Autodesk Inventor part; units mm, degrees
ref_plane "YZ Plane" through (0, 0, 0) normal (1, 0, 0) x (0, 1, 0)
ref_plane "XZ Plane" through (0, 0, 0) normal (0, 1, 0) x (-1, 0, 0)
ref_plane "XY Plane" through (0, 0, 0) normal (0, 0, 1) x (1, 0, 0)
sketch "Sketch1" plane through (0, 0, 0) normal (0, 0, 1) x (1, 0, 0)
  circle A0 centre (-18.3043, -1.4966) radius 1.7
  circle A1 centre (18.6957, -1.4966) radius 1.7
  circle A2 centre (18.6957, 6.5034) radius 1.7
  circle A3 centre (-18.3043, 6.5034) radius 1.7
  circle A4 centre (11.6957, 6.5034) radius 1.7
  arc A5 (22.6957, 8.5034) -> (18.6957, 12.5034) centre (18.6957, 8.5034) ccw
  line L0 (4.8957, 12.5034) -> (18.6957, 12.5034)
  arc A6 (4.8957, 12.5034) -> (2.8957, 10.5034) centre (4.8957, 10.5034) ccw
  line L1 (2.8957, 6.5034) -> (2.8957, 10.5034)
  arc A7 (-9.5043, 6.5034) -> (2.8957, 6.5034) centre (-3.3043, 6.5034) ccw
  line L2 (-9.5043, 10.5034) -> (-9.5043, 6.5034)
  arc A8 (-9.5043, 10.5034) -> (-11.5043, 12.5034) centre (-11.5043, 10.5034) ccw
  line L3 (-16.508, 12.5034) -> (-11.5043, 12.5034)
  line L4 (18.6957, -5.4966) -> (-18.3043, -5.4966)
  circle A9 centre (-18.3043, 6.5034) radius 1.7
  circle A10 centre (-26.3043, -2.4966) radius 1.6
  circle A11 centre (-26.3043, 15.5034) radius 1.6
  line L5 (-23.3147, 18.1609) -> (-16.508, 12.5034)
  arc A12 (-23.3147, 18.1609) -> (-30.3043, 15.5034) centre (-26.3043, 15.5034) ccw
  line L6 (-30.3043, 10.9756) -> (-30.3043, 15.5034)
  arc A13 (-30.3043, 10.9756) -> (-30.3043, 2.0313) centre (-26.3043, 6.5034) ccw
  line L7 (-30.3043, -2.4966) -> (-30.3043, 2.0313)
  arc A14 (-30.3043, -2.4966) -> (-27.7088, -6.2419) centre (-26.3043, -2.4966) ccw
  circle A15 centre (-26.3043, 6.5034) radius 2.5
  arc A16 (-18.3043, -5.4966) -> (-27.7088, -6.2419) centre (-19.7185, -47.358) ccw
  line L8 (22.6957, 8.5034) -> (22.6957, -1.4966)
  arc A17 (18.6957, -5.4966) -> (22.6957, -1.4966) centre (18.6957, -1.4966) ccw
  point P0 (0, 0)
  point P1 (-18.3043, 6.5034)
  dimension "d14" = 12
  dimension "d17" = 8
  dimension "d18" = 4
  dimension "d24" = 6
  dimension "d25" = 2
  dimension "d26" = 2
  dimension "d27" = 2
  dimension "d28" = 2
extrude "Extrusion1" add sketch "Sketch1" against normal blind 6
sketch "Sketch2" plane through (0, 0, -6) normal (0, 0, -1) x (-1, 0, 0)
  circle A0 centre (26.3043, -2.4966) radius 1.6
  circle A1 centre (26.3043, 15.5034) radius 1.6
  circle A2 centre (26.3043, 6.5034) radius 2.5
  arc A3 (30.3043, 15.5034) -> (23.3147, 18.1609) centre (26.3043, 15.5034) ccw
  circle A4 centre (18.3043, 6.5034) radius 1.7
  circle A5 centre (18.3043, -5.4966) radius 1.7
  circle A6 centre (26.3043, -2.4966) radius 1.6
  circle A7 centre (26.3043, 15.5034) radius 1.6
  line L0 (14.3043, 6.5034) -> (14.3043, -5.4966)
  arc A8 (14.3043, -5.4966) -> (19.7088, -9.2419) centre (18.3043, -5.4966) ccw
  line L1 (19.7088, -9.2419) -> (27.7088, -6.2419)
  arc A9 (27.7088, -6.2419) -> (30.3043, -2.4966) centre (26.3043, -2.4966) ccw
  line L2 (30.3043, -2.4966) -> (30.3043, 2.0313)
  arc A10 (30.3043, 2.0313) -> (30.3043, 10.9756) centre (26.3043, 6.5034) ccw
  line L3 (30.3043, 10.9756) -> (30.3043, 15.5034)
  arc A11 (30.3043, 15.5034) -> (23.3147, 18.1609) centre (26.3043, 15.5034) ccw
  line L4 (23.3147, 18.1609) -> (15.3147, 9.1609)
  arc A12 (15.3147, 9.1609) -> (14.3043, 6.5034) centre (18.3043, 6.5034) ccw
  line L5 (18.3043, 12.5242) -> (23.3147, 18.1609) construction
  arc A13 (27.7088, -6.2419) -> (18.3043, -5.4966) centre (19.7185, -47.358) ccw
  line L6 (23.3147, 18.1609) -> (16.508, 12.5034)
  line L7 (-4.8957, 12.5034) -> (-18.6957, 12.5034)
  line L8 (21.8043, 16.9055) -> (21.8043, -5.5246)
  line L9 (25.163, -7.1966) -> (21.8043, -5.5246)
  circle A14 centre (18.3043, 6.5034) radius 1.7
  point P0 (0, 0)
  dimension "d22" = 3.5
extrude "Extrusion2" add sketch "Sketch2" along normal blind 9 contours L3 A10 L2 A9 A13 L8 L4 A3 | L4 L8 L6
chamfer "Chamfer1" distance 1.5 angle 45 1 edges at (-21.8043, 5.6904, -6)
sketch "Sketch4" plane through (0, 0, -6) normal (0, 0, -1) x (-1, 0, 0)
  circle A0 centre (-11.6957, 6.5034) radius 1.7
  circle A1 centre (18.3043, 6.5034) radius 1.7
  line L0 (-8.4337, 6.5034) -> (-10.0647, 3.6784)
  line L1 (-10.0647, 3.6784) -> (-13.3267, 3.6784)
  line L2 (-13.3267, 3.6784) -> (-14.9577, 6.5034)
  line L3 (-14.9577, 6.5034) -> (-13.3267, 9.3284)
  line L4 (-13.3267, 9.3284) -> (-10.0647, 9.3284)
  line L5 (-10.0647, 9.3284) -> (-8.4337, 6.5034)
  line L6 (15.0423, 6.5034) -> (16.6733, 9.3284)
  line L7 (16.6733, 9.3284) -> (19.9353, 9.3284)
  line L8 (19.9353, 9.3284) -> (21.5663, 6.5034)
  line L9 (21.5663, 6.5034) -> (19.9353, 3.6784)
  line L10 (19.9353, 3.6784) -> (16.6733, 3.6784)
  line L11 (16.6733, 3.6784) -> (15.0423, 6.5034)
  dimension "d21" = 5.65
extrude "Extrusion3" cut sketch "Sketch4" against normal blind 3 and the other way blind 5
properties part number "Extruder_Fixer_BLTouch"
Check sheet for the modelled part. Datum: model origin and axes. Units: mm. A direction names the side the tool comes from. Give positions to 0.01 mm unless a question says otherwise; leave off trailing zeros. Loops run counter-clockwise (first coordinate to the right, second up) from the corner with the lowest first, then second, coordinate; pieces in that order, holes last. Notation, with made-up numbers: M 40,-32.5 L 68,-32.5 A15 cw 68,-24.5 Z; hole C 14.25,-5.75 d7. An arc over 180 degrees is marked long. Answer as a JSON object with one key per item and string values. Group by question number.
Q1. Release check for a two-part mould opening along Y. For faces 1 (the cylindrical face through (-20, -1.4, -3)), 2 (the cylindrical face through (21.49, -4.36, -2.96)), 3 (the cylindrical face through (21.555, 11.301, -2.958)), 4 (the flat face through (-9.504, 9, -3)) record: released by +Y, released by -Y, zero draft, split by the parting line, or undercut.
Q2. Cross-section at A-A on z = -1.75. Give the number of separate pieces and of enclosed holes in the cut face, then the cut area to 3 significant figures.
Q3. Go/stop test with flat-tipped pins: P1, Ø5.5, axis at x = -18.3, y = -1.5, coming from the +Z side; P2, Ø2, axis at y = 16, z = -6, coming from the +X side; P3, Ø4, axis at x = -14, z = -4.5, coming from the +Y side; P4, Ø2.5, axis at y = 0.5, z = -10.5, coming from the -X side. Record where each tip stops, or that it passes through.
Q4. Access from +Z, -Z, +X, -X, +Y, -Y to the whole of each face (thin tool, end or side, straight path). Record for faces 5 (the flat face through (22.696, 4, -3)), 6 (the flat face through (1, 1, -6)), 7 (the flat face through (14.15, 7.9, -4.52)), 8 (the cylindrical face through (17.347, 5.469, -2.958)), 9 (the cylindrical face through (3.497, 11.933, -2.958)).
Q5. Material ranges on line 1 along X through (y, z) = (4.75, -1); line 2 along X through (y, z) = (8.75, -1); line 3 along X through (y, z) = (7.5, -3.5), recorded low to high. Write a range as [from, to].
Q6. Cross-section at B-B on z = -13.25. Record the cut outline in (x, y), then the cut area to 3 significant figures.
Q7. Cross-section at C-C on y = 16.25. Record the cut outline in (x, z).
Q8. Cross-section at D-D on x = 17.5. Record the cut outline in (y, z), then the cut area to 3 significant figures.
Evaluation:
{
 "1": {"face 1": "undercut", "face 2": "released by -Y", "face 3": "released by +Y", "face 4": "zero draft"},
 "2": {"separate pieces": "1", "enclosed holes": "8", "area": "807 mm2"},
 "3": {"P1": "stops at z = 0", "P2": "stops at x = -19.51", "P3": "stops at y = 12.5", "P4": "stops at x = -30.3"},
 "4": {"face 5": "+Z, -Z, +X, +Y, -Y", "face 6": "-Z, +X, +Y, -Y", "face 7": "-Z", "face 8": "+Z, -Z", "face 9": "+Z, -Z, +Y"},
 "5": {"line 1": "x = [-32.04, -28.09], [-24.52, -9.25], [2.64, 22.7]", "line 2": "x = [-31.87, -27.4], [-25.21, -9.5], [2.9, 22.69]", "line 3": "x = [-32.22, -28.6], [-24.01, -20.99], [-15.62, -9.5], [2.9, 9.01], [14.38, 17.32], [20.07, 22.7]"},
 "6": {"outline": "M -30.3,-2.5 A4 ccw -27.71,-6.24 A41.88 cw -21.8,-5.52 L -21.8,16.91 L -23.31,18.16 A4 ccw -30.3,15.5 L -30.3,10.98 A6 ccw -30.3,2.03 Z; hole C -26.3,6.5 d5; hole C -26.3,-2.5 d3.2; hole C -26.3,15.5 d3.2", "area": "183 mm2"},
 "7": {"outline": "M -30.23,-15 L -27.72,-15 L -27.72,0 L -30.23,0 Z; M -24.89,-15 L -21.8,-15 L -21.8,-7.5 L -21.02,-6.71 L -21.02,0 L -24.89,0 Z"},
 "8": {"outline": "M -5.5,-6 L -2.71,-6 L -2.71,0 L -5.5,0 Z; M -0.29,-6 L 5.29,-6 L 5.29,0 L -0.29,0 Z; M 7.71,-6 L 12.5,-6 L 12.5,0 L 7.71,0 Z", "area": "79.0 mm2"}
}
